Input: part model. Units: mm. Frame: model coordinates. A direction names the side the tool comes from. Round coordinates to 2 decimals unless told otherwise and drop trailing zeros. Loops run counter-clockwise (first coordinate to the right, second up) from the corner with the lowest first, then second, coordinate; pieces in that order, holes last.
(1) First-contact query: pin 1 Ø8 at (x, z) = (-99.5, 39) entering from +Y; pin 2 Ø5 at (x, z) = (151.5, -19) entering from -Y; pin 3 Ø1 at (x, y) = (23, 769) entering from -Z. Flat tips, straight axial feed; report the tip coordinate or a pass-through.
(2) Draft query along X for faces 4 (the face through (-60, 622, 1)), 5 (the face through (50, 617, 1)), 6 (the face through (3, 0, -3)). Return one class per face: released by +X, released by -X, zero draft, split by the parting line, or undercut.
(3) Access query for faces 1 (the face through (-1, 622, 60)), 2 (the face through (-1, 622, -60)), 3 (the face through (3, 10, -3)). Directions: +Z, -Z, +X, -X, +Y, -Y. A direction counts if a zero-diameter tool reaches every point of the face in a straight line with its end or side. Return the directions, or none.
(4) Line query: line 1 (Y direction, x = -98, z = 77); line 2 (Z direction, x = 23.5, y = 638.5); line 3 (Y direction, x = -56.5, z = 37.5). Output: solid intervals per line, ascending.
(5) Cut plane B-B, the plane y = 981.5. Output: boundary loops of the cut face in (x, z), and give its area (3 significant figures).
from build123d import *

# Parameters (mm, degrees)
SKETCH1_R           = 200
BOSS_EXTRUDE1_DEPTH = 30
FILLET1_R           = 30
SKETCH2_W           = 120
SKETCH2_H           = 120
BOSS_EXTRUDE2_DEPTH = 1200
SHELL1_T            = -10


with BuildPart() as part:
    # Sketch1 → Boss-Extrude1 (new body)
    with BuildSketch(Plane(origin=(0, 0, 0), x_dir=(1, 0, 0), z_dir=(0, 1, 0))):
        with Locations(Location((0, 0, 0), (0, 0, 270))):
            Circle(SKETCH1_R)
    extrude(amount=BOSS_EXTRUDE1_DEPTH)

    # Fillet1
    fillet1_edges = [part.edges().sort_by_distance(p)[0] for p in [
        (0, 30, -200),
    ]]
    fillet(fillet1_edges, radius=FILLET1_R - 0.0001)  # a hair under: the kernel refuses the full size

    # Sketch2 → Boss-Extrude2 (add)
    with BuildSketch(Plane(origin=(0, 30, 0), x_dir=(1, 0, 0), z_dir=(0, 1, 0))):
        Rectangle(SKETCH2_W, SKETCH2_H)
    extrude(amount=BOSS_EXTRUDE2_DEPTH)

    # Shell1
    shell1_openings = [part.faces().sort_by_distance(p)[0] for p in [
        (0, 1230, 0),
    ]]
    offset(amount=SHELL1_T, openings=shell1_openings, kind=Kind.INTERSECTION)


solid = part.part
Reported:
1. pin 1: stops at y = 30
1. pin 2: stops at y = 0
1. pin 3: stops at z = -60
2. face 4: released by -X
2. face 5: undercut
2. face 6: zero draft
3. face 1: +Z, +X, -X, +Y
3. face 2: -Z, +X, -X, +Y
3. face 3: none
4. line 1: y = 0 to 10, 20 to 30
4. line 2: z = -60 to -50, 50 to 60
4. line 3: y = 0 to 10, 20 to 1230
5. outline: (-60, -60) - (60, -60) - (60, 60) - (-60, 60) - close; hole (-50, -50) - (50, -50) - (50, 50) - (-50, 50) - close
5. area: 4,400 mm2
